CAD build for the part. Positions are in the model's coordinates, mm. A direction names the side the tool comes from. Coordinates: 2 decimals unless noted, no trailing zeros. Loops run counter-clockwise (first coordinate to the right, second up) from the corner with the lowest first, then second, coordinate; pieces in that order, holes last. Notation, with made-up numbers: (25, 37) - (51, 37) arc R24 cw to (51, 62) - close; hole circle Ø4 at (20.5, -21.75). An arc over 180 degrees is marked (long way). Put each result on its own line as item: value.
```python
from build123d import *

# Parameters (mm, degrees)
BOSS_EXTRUDE1_DEPTH = 10
CUT_EXTRUDE1_DEPTH  = 6
SKETCH3_R           = 14
CUT_EXTRUDE2_DEPTH  = 100
SKETCH4_W           = 2.485456217
SKETCH4_H           = 52.416620737
CUT_EXTRUDE3_DEPTH  = 100


with BuildPart() as part:
    # Sketch1 → Boss-Extrude1 (new body)
    with BuildSketch(Plane.XY):
        with BuildLine():
            Line((-3.679977182, -54.534954407), (4.628170727, -54.534954407))
            Line((4.628170727, -54.534954407), (17.741392821, -45.792806344))
            Line((17.741392821, -45.792806344), (17.741392821, -11.427332251))
            Line((17.741392821, -11.427332251), (7.741392821, 3.572667749))
            Line((7.741392821, 3.572667749), (7.741392821, 103.024920211))
            ThreePointArc((7.741392821, 103.024920211), (-2.457335357, 112.462746672), (-12.242059824, 102.596349566))
            Line((-12.242059824, 102.596349566), (-12.242059824, 2.804284439))
            Line((-12.242059824, 2.804284439), (-22.364938744, -3.944301507))
            Line((-22.364938744, -3.944301507), (-22.364938744, -54.534954407))
            Line((-22.364938744, -54.534954407), (-3.679977182, -54.534954407))
        make_face()
        with BuildLine():
            Line((2.257078102, 102.465045593), (2.257078102, 12.465045593))
            ThreePointArc((2.257078102, 12.465045593), (-2.242921898, 7.965045593), (-6.742921898, 12.465045593))
            Line((-6.742921898, 12.465045593), (-6.742921898, 102.465045593))
            ThreePointArc((-6.742921898, 102.465045593), (-2.242921898, 106.965045593), (2.257078102, 102.465045593))
        make_face(mode=Mode.SUBTRACT)
    extrude(amount=BOSS_EXTRUDE1_DEPTH)

    # Sketch2 → Cut-Extrude1 (cut)
    with BuildSketch(Plane.XY.offset(10)):
        with BuildLine():
            Line((4.757078102, 102.465045593), (4.757078102, 9.430262407))
            ThreePointArc((4.757078102, 9.430262407), (-2.242921898, 2.430262407), (-9.242921898, 9.430262407))
            Line((-9.242921898, 9.430262407), (-9.242921898, 102.465045593))
            ThreePointArc((-9.242921898, 102.465045593), (-2.242921898, 109.465045593), (4.757078102, 102.465045593))
        make_face()
    extrude(amount=-CUT_EXTRUDE1_DEPTH, mode=Mode.SUBTRACT)

    # Sketch3 → Cut-Extrude2 (cut)
    with BuildSketch(Plane.XY.offset(10)):
        with Locations((0, -24.534954407)):
            Circle(SKETCH3_R)
    extrude(amount=-CUT_EXTRUDE2_DEPTH, mode=Mode.SUBTRACT)

    # Sketch4 → Cut-Extrude3 (cut)
    with BuildSketch(Plane.XY.offset(10)):
        with Locations((-1.385400928, -52.416791412)):
            Rectangle(SKETCH4_W, SKETCH4_H)
    extrude(amount=-CUT_EXTRUDE3_DEPTH, mode=Mode.SUBTRACT)


solid = part.part
```
Q1. Wall check: L1, parallel to X at y = 102, z = 2; L2, parallel to Y at x = 0.5, z = 3.75; L3, parallel to X at y = 83, z = 7.5. Give the ranges that are in metal, low to high. Write a range as from..to.
Determined:
L1: -12.24..-6.74, 2.26..7.74
L2: -54.53..-38.53, -10.54..8.9, 106.03..112.08
L3: -12.24..-9.24, 4.76..7.74
Q2. Mould opens along Y. For faces 1 (the flat face through (-2.628, -47, 5)), 2 (the flat face through (2.257, 58, 2)), 3 (the flat face through (12.81, -4.03, 4.93)) say: +Y half, -Y half, draft (parallel to the pull), parting line (faces both ways), or undercut.
Determined:
face 1: draft
face 2: undercut
face 3: +Y half
Q3. Pin check, flat tips, straight feed: pin 1 Ø22.5 at (x, y) = (0, -24.53) entering from +Z; pin 2 Ø3 at (y, z) = (67, 7) entering from -X; pin 3 Ø2 at (y, z) = (65, 1.5) entering from +X; pin 4 Ø1.5 at (x, z) = (5.5, 4) entering from +Y. Stop position of each tip, or through.
Determined:
pin 1: through
pin 2: x = -12.24
pin 3: x = 7.74
pin 4: y = 109.61
Q4. Slice it at A-A, the plane z = 5.5. Give the cut face in (x, y).
Determined:
outline: (-22.36, -54.53) - (-2.63, -54.53) - (-2.63, -38.29) arc R14 cw (long way) to (-0.14, -38.53) - (-0.14, -54.53) - (4.63, -54.53) - (17.74, -45.79) - (17.74, -11.43) - (7.74, 3.57) - (7.74, 103.02) arc R10 ccw to (-12.24, 102.6) - (-12.24, 2.8) - (-22.36, -3.94) - close; hole (-9.24, 9.43) arc R7 ccw to (4.76, 9.43) - (4.76, 102.47) arc R7 ccw to (-9.24, 102.47) - close
Q5. Tool access for faces 4 (the flat face through (3, 57, 4)), 5 (the cylindrical face through (-2.144, 7.966, 1.972)), 6 (the flat face through (-12.242, 53, 5)): list every direction of +Z, -Z, +X, -X, +Y, -Y with a clear straight run to the whole face (end or side of a thin tool).
Determined:
face 4: +Z
face 5: +Z, -Z
face 6: +Z, -Z, -X, +Y
